from build123d import *

# Parameters (mm, degrees)
CROQUIS1_W              = 68
CROQUIS1_H              = 60
CROQUIS1_R              = 1.5
SALIENTE_EXTRUIR2_DEPTH = 3
CROQUIS2_W              = 5
CROQUIS2_H              = 10
SALIENTE_EXTRUIR3_DEPTH = 13
CORTAR_EXTRUIR1_DEPTH   = 13
CROQUIS4_R              = 1.5
CORTAR_EXTRUIR2_DEPTH   = 13
CROQUIS6_W              = 0.75
CROQUIS6_H              = 19.11
CROQUIS6_H_2            = 18.27
CORTAR_EXTRUIR3_DEPTH   = 10
CROQUIS7_W              = 7.48396125
CROQUIS7_H              = 18.688270588
CORTAR_EXTRUIR4_DEPTH   = 10
CROQUIS8_W              = 10
CROQUIS8_H              = 10
SALIENTE_EXTRUIR4_DEPTH = 13
CROQUIS9_W              = 60
CROQUIS9_H              = 30
SALIENTE_EXTRUIR5_DEPTH = 3
CROQUIS10_R             = 4.25
CORTAR_EXTRUIR5_DEPTH   = 3
REDONDEO1_R             = 5


with BuildPart() as part:
    # Croquis1 → Saliente-Extruir2 (new body)
    with BuildSketch(Plane(origin=(0, 0, 0), x_dir=(1, 0, 0), z_dir=(0, 1, 0))):
        Rectangle(CROQUIS1_W, CROQUIS1_H)
        with Locations(Location((-29, 25, 0), (0, 0, 270))):
            Circle(CROQUIS1_R, mode=Mode.SUBTRACT)
        with Locations(Location((29, 25, 0), (0, 0, 270))):
            Circle(CROQUIS1_R, mode=Mode.SUBTRACT)
        with Locations(Location((-29, -25, 0), (0, 0, 270))):
            Circle(CROQUIS1_R, mode=Mode.SUBTRACT)
        with Locations(Location((29, -25, 0), (0, 0, 270))):
            Circle(CROQUIS1_R, mode=Mode.SUBTRACT)
    extrude(amount=SALIENTE_EXTRUIR2_DEPTH)

    # Croquis2 → Saliente-Extruir3 (add)
    with BuildSketch(Plane(origin=(0, 3, 0), x_dir=(1, 0, 0), z_dir=(0, 1, 0))):
        Rectangle(CROQUIS2_W, CROQUIS2_H)
    extrude(amount=SALIENTE_EXTRUIR3_DEPTH)

    # Croquis3 → Cortar-Extruir1 (cut)
    with BuildSketch(Plane(origin=(2.5, 0, 0), x_dir=(0, 0, -1), z_dir=(1, 0, 0))):
        with BuildLine():
            Line((-5, 16), (-5, 11))
            ThreePointArc((-5, 11), (-3.535533906, 14.535533906), (0, 16))
            Line((0, 16), (-5, 16))
        make_face()
        with BuildLine():
            ThreePointArc((0, 16), (3.535533906, 14.535533906), (5, 11))
            Line((5, 11), (5, 16))
            Line((5, 16), (0, 16))
        make_face()
    extrude(amount=-CORTAR_EXTRUIR1_DEPTH, mode=Mode.SUBTRACT)

    # Croquis4 → Cortar-Extruir2 (cut)
    with BuildSketch(Plane(origin=(2.5, 0, 0), x_dir=(0, 0, -1), z_dir=(1, 0, 0))):
        with Locations((0, 11)):
            Circle(CROQUIS4_R)
    extrude(amount=-CORTAR_EXTRUIR2_DEPTH, mode=Mode.SUBTRACT)

    # Croquis6 → Cortar-Extruir3 (cut)
    with BuildSketch(Plane(origin=(0, 0, -5), x_dir=(-1, 0, 0), z_dir=(0, 0, -1))):
        with Locations((-2.125, 12.555)):
            Rectangle(CROQUIS6_W, CROQUIS6_H)
        with Locations((2.125, 12.135)):
            Rectangle(CROQUIS6_W, CROQUIS6_H_2)
    extrude(amount=-CORTAR_EXTRUIR3_DEPTH, mode=Mode.SUBTRACT)

    # Croquis7 → Cortar-Extruir4 (cut)
    with BuildSketch(Plane(origin=(0, 0, -5), x_dir=(-1, 0, 0), z_dir=(0, 0, -1))):
        with Locations((1.991980625, 12.344135294)):
            Rectangle(CROQUIS7_W, CROQUIS7_H)
    extrude(amount=-CORTAR_EXTRUIR4_DEPTH, mode=Mode.SUBTRACT)

    # Croquis8 → Saliente-Extruir4 (add)
    with BuildSketch(Plane(origin=(0, 3, 0), x_dir=(1, 0, 0), z_dir=(0, 1, 0))):
        Rectangle(CROQUIS8_W, CROQUIS8_H)
    extrude(amount=SALIENTE_EXTRUIR4_DEPTH)

    # Croquis9 → Saliente-Extruir5 (add)
    with BuildSketch(Plane(origin=(0, 16, 0), x_dir=(1, 0, 0), z_dir=(0, 1, 0))):
        Rectangle(CROQUIS9_W, CROQUIS9_H)
    extrude(amount=SALIENTE_EXTRUIR5_DEPTH)

    # Croquis10 → Cortar-Extruir5 (cut)
    with BuildSketch(Plane(origin=(0, 19, 0), x_dir=(1, 0, 0), z_dir=(0, 1, 0))):
        with Locations(Location((-15, 0, 0), (0, 0, 270))):
            Circle(CROQUIS10_R)
        with Locations(Location((15, 0, 0), (0, 0, 270))):
            Circle(CROQUIS10_R)
    extrude(amount=-CORTAR_EXTRUIR5_DEPTH, mode=Mode.SUBTRACT)

    # Redondeo1
    redondeo1_edges = [part.edges().sort_by_distance(p)[0] for p in [
        (30, 17.5, 15),
        (30, 17.5, -15),
        (-30, 17.5, -15),
        (-30, 17.5, 15),
    ]]
    fillet(redondeo1_edges, radius=REDONDEO1_R)


solid = part.part
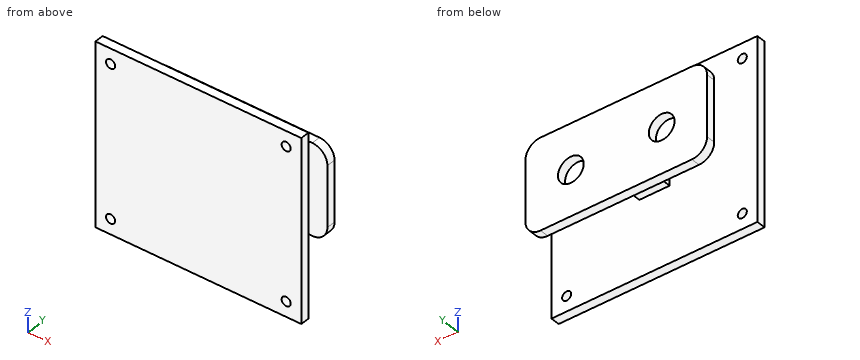
Input: part model. Units: mm. Frame: model coordinates. Coordinates: 2 decimals unless noted, no trailing zeros. Loops run counter-clockwise (first coordinate to the right, second up) from the corner with the lowest first, then second, coordinate; pieces in that order, holes last. Notation, with made-up numbers: (39, -11.5) - (78, -11.5) arc R20 cw to (78, 12.5) - close; hole circle Ø5 at (2, -10.75). An arc over 180 degrees is marked (long way). Answer in a Markdown table with one row per item. Add a question column.
Item 1: Section query B-B on x = 15. Return the cut outline in (y, z).
Item 2: Contact query for flat-ended pins moving along their axis: P1, Ø6, axis at x = 1, y = 9.5, coming from the -Z side; P2, Ø7.5, axis at x = -15, z = 0, coming from the +Y side; P3, Ø3, axis at x = 0, y = 11.5, coming from the +Z side. Output: stop coordinate, or through.
Item 3: Section query D-D on x = -29. Return the cut outline in (y, z), then the cut area to 3 significant figures.
Item 4: Line query: line 1 along X through (y, z) = (2.25, -25); line 2 along X through (y, z) = (16.8, 0); line 3 along Y through (x, z) = (2.5, -13). Output: solid intervals per line, ascending. Write a range as [from, to].
Item 5: Section query A-A on x = 7.5. Return the cut outline in (y, z), then the cut area to 3 significant figures.
Item 6: Section query C-C on z = -25. Return the cut outline in (x, y), then the cut area to 3 significant figures.
Recorded:
| question | item | result |
|---|---|---|
| 1 | outline | (0, -30) - (3, -30) - (3, 30) - (0, 30) - close; (16, -15) - (19, -15) - (19, -4.25) - (16, -4.25) - close; (16, 4.25) - (19, 4.25) - (19, 15) - (16, 15) - close |
| 2 | P1 | z = -5 |
| 2 | P2 | y = 3 |
| 2 | P3 | z = 5 |
| 3 | outline | (0, -30) - (3, -30) - (3, -26.5) - (0, -26.5) - close; (0, -23.5) - (3, -23.5) - (3, 23.5) - (0, 23.5) - close; (0, 26.5) - (3, 26.5) - (3, 30) - (0, 30) - close; (16, -13) - (19, -13) - (19, 13) - (16, 13) - close |
| 3 | area | 240 mm^2 |
| 4 | line 1 | [-34, -30.5], [-27.5, 27.5], [30.5, 34] |
| 4 | line 2 | [-30, -19.25], [-10.75, 10.75], [19.25, 30] |
| 4 | line 3 | [0, 3], [16, 19] |
| 5 | outline | (0, -30) - (3, -30) - (3, 30) - (0, 30) - close; (16, -15) - (19, -15) - (19, 15) - (16, 15) - close |
| 5 | area | 270 mm^2 |
| 6 | outline | (-34, 0) - (-30.5, 0) - (-30.5, 3) - (-34, 3) - close; (-27.5, 0) - (27.5, 0) - (27.5, 3) - (-27.5, 3) - close; (30.5, 0) - (34, 0) - (34, 3) - (30.5, 3) - close |
| 6 | area | 186 mm^2 |
